The listing builds one solid part. Answer for the finished solid, in the listing's coordinates (mm). Coordinates: 2 decimals unless noted, no trailing zeros. Loops run counter-clockwise (first coordinate to the right, second up) from the corner with the lowest first, then second, coordinate; pieces in that order, holes last. Notation, with made-up numbers: M 84,-23.5 L 96,-23.5 A13 ccw 96,-6.5 Z; hole C -34,-32.5 d5. An arc over 180 degrees is marked long. Return JSON: item names as keys, results as strings. Group by question number.
1. Section C-C (x = -14) is taken. Write down the section's boundary in (y, z), then the cut area to 3 significant figures.
2. Given P1, Ø2, axis at x = 153.5, y = 5, coming from the +Z side; P2, Ø1, axis at y = 1.5, z = 37, coming from the -X side; P3, Ø2.5, axis at x = -19.5, y = 5.5, coming from the +Z side, each flat-ended and moving along its own axis, determine where each tip first touches the part or whether it passes through.
3. Section D-D (z = 0) is taken. Write down the section's boundary in (x, y), then the cut area to 3 significant figures.
4. Section A-A (z = 40) is taken. Write down the section's boundary in (x, y), then the cut area to 3 significant figures.
5. Section B-B (y = 2.5) is taken. Write down the section's boundary in (x, z).
6. Straight lines are drawn through the part: L1, parallel to X at y = 6, z = 40.5; L2, parallel to Z at x = 58, y = 2.75; L3, parallel to X at y = 7, z = 23.5. For each, find the intervals that lie inside material, in ascending order. Write a range as from..to.
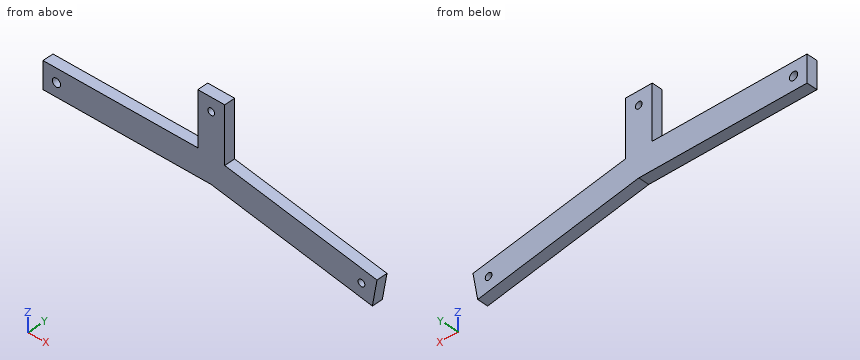
```python
from build123d import *

# Parameters (mm, degrees)
SKETCH1_R           = 3.05
SKETCH1_R_2         = 2.5
BOSS_EXTRUDE1_DEPTH = 8


with BuildPart() as part:
    # Sketch1 → Boss-Extrude1 (new body)
    with BuildSketch(Plane(origin=(0, 0, 0), x_dir=(1, 0, 0), z_dir=(0, 1, 0))):
        Polygon((75.861805451, 10), (195.542164518, 31.102876365), (199.018293649, 11.388768424), (85.861805451, -8.263285294), (85.861805451, -50), (75.861805451, -50), (65.861805451, -50), (65.861805451, -10), (-49.138194549, -10), (-49.138194549, 10), align=None)
        with Locations(Location((-39.138194549, 0, 0), (0, 0, 270))):
            Circle(SKETCH1_R, mode=Mode.SUBTRACT)
        with Locations(Location((75.861805451, -40, 0), (0, 0, 270))):
            Circle(SKETCH1_R_2, mode=Mode.SUBTRACT)
        with Locations(Location((187.432151553, 19.509340618, 0), (0, 0, 270))):
            Circle(SKETCH1_R_2, mode=Mode.SUBTRACT)
    extrude(amount=BOSS_EXTRUDE1_DEPTH)


solid = part.part
```
Worked out:
{
 "1": {"outline": "M 0,-10 L 8,-10 L 8,10 L 0,10 Z", "area": "160 mm^2"},
 "2": {"P1": "z = -3.31", "P2": "x = 65.86", "P3": "z = 10"},
 "3": {"outline": "M -49.14,0 L -42.19,0 L -42.19,8 L -49.14,8 Z; M -36.09,0 L 133.44,0 L 133.44,8 L -36.09,8 Z", "area": "1,410 mm^2"},
 "4": {"outline": "M 65.86,0 L 73.36,0 L 73.36,8 L 65.86,8 Z; M 78.36,0 L 85.86,0 L 85.86,8 L 78.36,8 Z", "area": "120 mm^2"},
 "5": {"outline": "M -49.14,-10 L 75.86,-10 L 195.54,-31.1 L 199.02,-11.39 L 85.86,8.26 L 85.86,50 L 65.86,50 L 65.86,10 L -49.14,10 Z; hole C -39.14,0 d6.1; hole C 75.86,40 d5; hole C 187.43,-19.51 d5"},
 "6": {"L1": "65.86..73.41, 78.31..85.86", "L2": "-10..10", "L3": "65.86..85.86"}
}
